The listing builds one solid part. Answer for the finished solid, in the listing's coordinates (mm). Round coordinates to 2 decimals unless told otherwise and drop trailing zeros.
(1) Find the intervals of material crossed by probe 1 along Z at (x, y) = (2.25, 5.5) (3 decimals); probe 2 along Z at (x, y) = (13, 20.25) (3 decimals); probe 3 along Z at (x, y) = (7, 10) (3 decimals), in increasing order.
(2) A cutting plane is placed at A-A, the plane y = 11.5. Give the number of separate pieces and of enclosed holes in the cut face, and give its area (3 significant figures).
(3) The mould has two halves that part along Z. Classify faces 1 (the face through (8, 13, 0)), 2 (the face through (13.07, 12.87, 56.1)), 3 (the face through (7.077, 12.867, 113.412)), 4 (the face through (14, 25.4, 58)): +Z half, -Z half, draft (parallel to the pull), parting line (faces both ways), or undercut.
Autodesk Inventor part; units mm, degrees
ref_plane "YZ Plane" through (0, 0, 0) normal (1, 0, 0) x (0, 1, 0)
ref_plane "XZ Plane" through (0, 0, 0) normal (0, 1, 0) x (-1, 0, 0)
ref_plane "XY Plane" through (0, 0, 0) normal (0, 0, 1) x (1, 0, 0)
sketch "Sketch1" plane through (0, 0, 0) normal (0, 0, 1) x (1, 0, 0)
  line L0 (0, 0) -> (15.875, 0)
  line L1 (15.875, 0) -> (15.875, 25.4)
  line L2 (15.875, 25.4) -> (0, 25.4)
  line L3 (0, 25.4) -> (0, 0)
  dimension "d0" = 15.875
  dimension "d1" = 25.4
extrude "Extrusion1" add sketch "Sketch1" along normal blind 117.475
chamfer "Chamfer1" distance 0.762 angle 45 11 edges at (15.875, 25.4, 58.7375) (7.9375, 25.4, 117.475) (0, 25.4, 58.7375) (7.9375, 25.4, 0) (15.875, 12.7, 0) (15.875, 0, 58.7375) (0, 12.7, 0) (0, 0, 58.7375) (15.875, 12.7, 117.475) (0, 12.7, 117.475) (7.9375, 0, 117.475)
sketch "Sketch2" plane through (0.762, 25.4, 0.762) normal (0, 1, 0) x (1, 0, 0)
  line L0 (14.351, 0.762) -> (0, 0.762)
  line L1 (0, -116.713) -> (14.351, -116.713)
  line L2 (-0.762, 0) -> (-0.762, -115.951)
  line L3 (15.113, -115.951) -> (15.113, 0)
  circle A0 centre (7.1755, -108.7755) radius 3.9688
  circle A1 centre (7.1755, -70.6755) radius 3.175
  circle A2 centre (7.1755, -53.213) radius 5.5563
  circle A3 centre (7.1755, -7.1755) radius 3.9688
  point P0 (-0.762, 0.762)
  dimension "d7" = 7.9375
  dimension "d8" = 7.9375
  dimension "d9" = 71.4375
  dimension "d10" = 53.975
  dimension "d11" = 7.9375
  dimension "d12" = 7.9375
  dimension "d13" = 6.35
  dimension "d14" = 11.1125
  dimension "d15" = 7.9375
extrude "Extrusion2" cut sketch "Sketch2" against normal blind 117.475
sketch "Sketch3" plane through (15.875, 0.762, 0.762) normal (1, 0, 0) x (0, 0, -1)
  line L0 (0.762, -0.762) -> (0.762, 23.876)
  line L1 (-115.951, -0.762) -> (0.762, -0.762)
  circle A0 centre (-40.513, 16.7005) radius 3.175
  circle A1 centre (-26.2255, 4.8006) radius 2.3813
  dimension "d18" = 26.9875
  dimension "d19" = 5.5626
  dimension "d20" = 17.4625
  dimension "d21" = 41.275
  dimension "d22" = 6.35
  dimension "d23" = 4.7625
extrude "Extrusion3" cut sketch "Sketch3" against normal blind 117.475
chamfer "Chamfer2" distance 0.762 angle 45 11 edges at (2.3812, 25.4, 53.975) (4.7625, 25.4, 71.4375) (3.9687, 25.4, 109.5375) (3.9687, 25.4, 7.9375) (15.875, 17.4625, 44.45) (15.875, 5.5626, 29.3688) (7.9375, 0, 0) (3.9687, 0, 7.9375) (2.3812, 0, 53.975) (4.7625, 0, 71.4375) (3.9687, 0, 109.5375)
properties part number "Upper Die Center Support"
Solutions:
1. probe 1: z = 0 to 24.607, 29.368 to 117.475
1. probe 2: z = 0 to 39.755, 42.795 to 51.685, 56.265 to 117.475
1. probe 3: z = 0 to 4.081, 11.794 to 48.498, 59.452 to 68.404, 74.471 to 105.681, 113.394 to 117.475
2. separate pieces: 1
2. enclosed holes: 4
2. area: 1,640 mm2
3. face 1: -Z half
3. face 2: undercut
3. face 3: undercut
3. face 4: draft
